Design review of the part built by this model. Coordinates are the model's own, in mm. A direction names the side the tool comes from. Give positions to 0.01 mm unless a question says otherwise; leave off trailing zeros. Order: outer loops, then holes, each group sorted by start corner. A loop starts at its lowest first (then second) coordinate and runs counter-clockwise, first axis right, second up. Notation, with made-up numbers: (65.25, -11.5) -> (102.25, -11.5) arc R20 ccw to (102.25, 12.5) -> close; hole circle Ø2 at (-23.75, -32.5). An arc over 180 degrees is marked (long way). Return JSON: item names as keys, results as strings.
```python
from build123d import *

# Parameters (mm, degrees)
SKETCH1_W           = 10.5
SKETCH1_H           = 10
BOSS_EXTRUDE1_DEPTH = 7.5
SHELL1_T            = 1
CUT_EXTRUDE1_REACH  = 12.431
SKETCH2_R           = 3.85
SKETCH3_W           = 8.5
SKETCH3_H           = 8
CUT_EXTRUDE2_DEPTH  = 1


with BuildPart() as part:
    # Sketch1 → Boss-Extrude1 (new body)
    with BuildSketch(Plane.XY):
        Rectangle(SKETCH1_W, SKETCH1_H)
    extrude(amount=BOSS_EXTRUDE1_DEPTH)

    # Shell1 (no face opened: a closed hollow body)
    add(offset(amount=-SHELL1_T, mode=Mode.PRIVATE), mode=Mode.SUBTRACT)

    # Sketch2 → Cut-Extrude1 (cut, up to next)
    with BuildSketch(Plane.XY.offset(7.5), mode=Mode.PRIVATE) as cut_extrude1_sk1:
        Circle(SKETCH2_R)
    cut_extrude1_tool1 = extrude(cut_extrude1_sk1.sketch, amount=-CUT_EXTRUDE1_REACH, mode=Mode.PRIVATE) & part.part
    add(cut_extrude1_tool1.solids().sort_by_distance((0, 0, 7.5))[0], mode=Mode.SUBTRACT)

    # Sketch3 → Cut-Extrude2 (cut)
    with BuildSketch(Plane.XY):
        Rectangle(SKETCH3_W, SKETCH3_H)
    extrude(amount=CUT_EXTRUDE2_DEPTH, mode=Mode.SUBTRACT)


solid = part.part
```
Item 1: Mouldability with a two-part tool opening along Y and no side actions: class faces 3 (the face through (2.3, 3.4, 7.5)), 4 (the face through (0, 4, 3)), 5 (the face through (-3, 3, 6.5)), 6 (the face through (0, 5, 4)) as released by +Y, released by -Y, zero draft, split by the parting line, or undercut.
Result set:
{"face 3": "zero draft", "face 4": "undercut", "face 5": "undercut", "face 6": "released by +Y"}
Item 2: Add section A-A (z = 3.5). Give the boundary of the cut face in (x, y), plus the area to 3 significant figures.
Result set:
{"outline": "(-5.25, -5) -> (5.25, -5) -> (5.25, 5) -> (-5.25, 5) -> close; hole (-4.25, -4) -> (4.25, -4) -> (4.25, 4) -> (-4.25, 4) -> close", "area": "37.0 mm^2"}
Item 3: Wall thickness on L1, parallel to Y at x = 0, z = 7.1; L2, parallel to X at y = 1.5, z = 0.5; L3, parallel to Y at x = -0.75, z = 0.75: over which ranges is each line inside the solid? List them lowest first. Write a range as [from, to].
Result set:
{"L1": "y = [-5, -3.85], [3.85, 5]", "L2": "x = [-5.25, -4.25], [4.25, 5.25]", "L3": "y = [-5, -4], [4, 5]"}
Item 4: Add section B-B (y = -2). Give the boundary of the cut face in (x, z), plus the area to 3 significant figures.
Result set:
{"outline": "(-5.25, 0) -> (-4.25, 0) -> (-4.25, 6.5) -> (-3.29, 6.5) -> (-3.29, 7.5) -> (-5.25, 7.5) -> close; (3.29, 6.5) -> (4.25, 6.5) -> (4.25, 0) -> (5.25, 0) -> (5.25, 7.5) -> (3.29, 7.5) -> close", "area": "16.9 mm^2"}
Item 5: Add section C-C (x = 0). Give the boundary of the cut face in (y, z), plus the area to 3 significant figures.
Result set:
{"outline": "(-5, 0) -> (-4, 0) -> (-4, 6.5) -> (-3.85, 6.5) -> (-3.85, 7.5) -> (-5, 7.5) -> close; (3.85, 6.5) -> (4, 6.5) -> (4, 0) -> (5, 0) -> (5, 7.5) -> (3.85, 7.5) -> close", "area": "15.3 mm^2"}
Item 6: Machinability: for faces 1 (the face through (0, -5, 4)), 2 (the face through (0, -4, 3)), which of the approach directions +Z, -Z, +X, -X, +Y, -Y give a long, thin tool a straight path to every point of the face, cutting with its end or side? Answer none if there is none.
Result set:
{"face 1": "+Z, -Z, +X, -X, -Y", "face 2": "-Z"}
